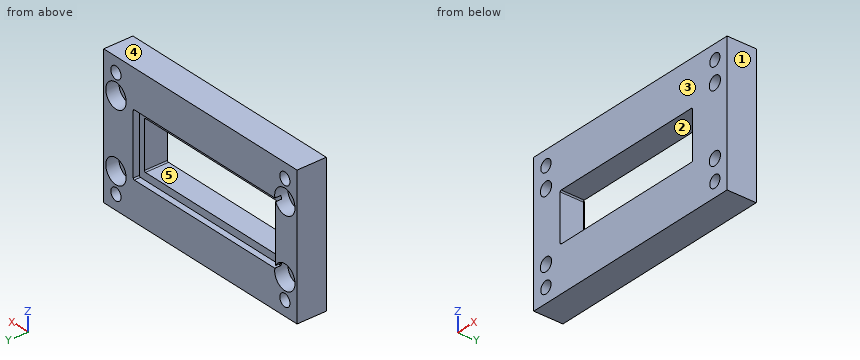
from build123d import *

# Parameters (mm, degrees)
SKETCH1_W                                   = 95
SKETCH1_H                                   = 57
SKETCH1_R                                   = 2.057983022
BOSS_EXTRUDE2_DEPTH                         = 12
BOSS_EXTRUDE3_DEPTH                         = 9.5
CBORE_FOR_M6_CHEESE_HEAD_SCREW1_D           = 5.5
CBORE_FOR_M6_CHEESE_HEAD_SCREW1_CBORE_D     = 10
CBORE_FOR_M6_CHEESE_HEAD_SCREW1_CBORE_DEPTH = 5.4
F_5_0_5_DIAMETER_HOLE1_D                    = 5


with BuildPart() as part:
    # Sketch1 → Boss-Extrude2 (new body)
    with BuildSketch(Plane(origin=(0, 0, 0), x_dir=(1, 0, 0), z_dir=(0, 1, 0))):
        Rectangle(SKETCH1_W, SKETCH1_H)
        with Locations(Location((41.5, 22.5, 0), (0, 0, 270))):
            Circle(SKETCH1_R, mode=Mode.SUBTRACT)
        with Locations(Location((-41.5, 22.5, 0), (0, 0, 270))):
            Circle(SKETCH1_R, mode=Mode.SUBTRACT)
        with Locations(Location((41.5, -22.5, 0), (0, 0, 270))):
            Circle(SKETCH1_R, mode=Mode.SUBTRACT)
        with Locations(Location((-41.5, -22.5, 0), (0, 0, 270))):
            Circle(SKETCH1_R, mode=Mode.SUBTRACT)
        with BuildLine():
            Line((-37, 12.5), (-37, -12.5))
            ThreePointArc((-37, -12.5), (-36.853553391, -12.853553391), (-36.5, -13))
            Line((-36.5, -13), (32.5, -13))
            ThreePointArc((32.5, -13), (32.853553391, -12.853553391), (33, -12.5))
            Line((33, -12.5), (33, 12.5))
            ThreePointArc((33, 12.5), (32.853553391, 12.853553391), (32.5, 13))
            Line((32.5, 13), (-36.5, 13))
            ThreePointArc((-36.5, 13), (-36.853553391, 12.853553391), (-37, 12.5))
        make_face(mode=Mode.SUBTRACT)
    extrude(amount=BOSS_EXTRUDE2_DEPTH)

    # Sketch1_5 → Boss-Extrude3 (add)
    with BuildSketch(Plane(origin=(0, 0, 0), x_dir=(1, 0, 0), z_dir=(0, 1, 0))):
        with BuildLine():
            ThreePointArc((-37, 12.5), (-36.853553391, 12.853553391), (-36.5, 13))
            Line((-36.5, 13), (32.5, 13))
            ThreePointArc((32.5, 13), (32.853553391, 12.853553391), (33, 12.5))
            Line((33, 12.5), (33, -12.5))
            ThreePointArc((33, -12.5), (32.853553391, -12.853553391), (32.5, -13))
            Line((32.5, -13), (-36.5, -13))
            ThreePointArc((-36.5, -13), (-36.853553391, -12.853553391), (-37, -12.5))
            Line((-37, -12.5), (-37, 12.5))
        make_face()
        with BuildLine():
            ThreePointArc((30, -10), (30.353553391, -9.853553391), (30.5, -9.5))
            Line((30.5, -9.5), (30.5, 9.5))
            ThreePointArc((30.5, 9.5), (30.353553391, 9.853553391), (30, 10))
            Line((30, 10), (-34, 10))
            ThreePointArc((-34, 10), (-34.353553391, 9.853553391), (-34.5, 9.5))
            Line((-34.5, 9.5), (-34.5, -9.5))
            ThreePointArc((-34.5, -9.5), (-34.353553391, -9.853553391), (-34, -10))
            Line((-34, -10), (30, -10))
        make_face(mode=Mode.SUBTRACT)
    extrude(amount=BOSS_EXTRUDE3_DEPTH)

    # CBORE for M6 Cheese Head Screw1 (through all)
    with Locations(Plane(origin=(-41.5, 12, -14), x_dir=(0, 0, 1), z_dir=(0, 1, 0))):
        with Locations((0, 0), (0, 83), (28, 83), (28, 0)):
            CounterBoreHole(CBORE_FOR_M6_CHEESE_HEAD_SCREW1_D / 2, CBORE_FOR_M6_CHEESE_HEAD_SCREW1_CBORE_D / 2, CBORE_FOR_M6_CHEESE_HEAD_SCREW1_CBORE_DEPTH)

    # 5.0 _5_ Diameter Hole1 (through all)
    with Locations(Plane(origin=(-41.5, 12, -22.5), x_dir=(0, 0, 1), z_dir=(0, 1, 0))):
        with Locations((0, 0), (0, 83), (45, 83), (45, 0)):
            Hole(F_5_0_5_DIAMETER_HOLE1_D / 2)


solid = part.part
The listing builds one solid part. Answer for the finished solid, in the listing's coordinates (mm). Face numbers are marked on the shaded views. A direction names the side the tool comes from. Give positions to 0.01 mm unless a question says otherwise; leave off trailing zeros. Write each loop counter-clockwise with the first axis right and the second up, starting at its lowest first coordinate (ties: lowest second). Pieces come first, ordered by that corner, then holes. Notation, with made-up numbers: (6, 53) - (46, 53) arc R14 ccw to (46, 79) - close; hole circle Ø8 at (6.5, 7.5). An arc over 180 degrees is marked (long way). Use a Markdown table: item, result.
1. Section D-D on x = -3.5 is taken. Write down the section's boundary in (y, z).
Values follow:
| item | result |
|---|---|
| outline | (0, -28.5) - (12, -28.5) - (12, -13) - (9.5, -13) - (9.5, -10) - (0, -10) - close; (0, 10) - (9.5, 10) - (9.5, 13) - (12, 13) - (12, 28.5) - (0, 28.5) - close |
2. Each of these flat-tipped pins is pushed along its axis until it touches: P1, Ø7, axis at x = -41.5, z = -14, coming from the -Y side; P2, Ø8, axis at x = 41.5, z = 14, coming from the +Y side. Where does it stop, or does it pass through?
Values follow:
| item | result |
|---|---|
| P1 | stops at y = 0 |
| P2 | stops at y = 6.6 |
3. Section A-A on z = -22.5 is taken. Write down the section's boundary in (x, y), plus the area to 3 significant figures.
Values follow:
| item | result |
|---|---|
| outline | (-47.5, 0) - (-44, 0) - (-44, 12) - (-47.5, 12) - close; (-39, 0) - (39, 0) - (39, 12) - (-39, 12) - close; (44, 0) - (47.5, 0) - (47.5, 12) - (44, 12) - close |
| area | 1,020 mm² |
4. For a pull along X with two mould halves and no side action, classify the marked faces 1, 2 and 3 as released by +X, released by -X, zero draft, split by the parting line, or undercut.
Values follow:
| item | result |
|---|---|
| face 1 | released by +X |
| face 2 | undercut |
| face 3 | zero draft |
5. Find the intervals of material crossed by probe 1 along X at (y, z) = (6.25, 22.5); probe 2 along X at (y, z) = (8.1, 14); probe 3 along Z at (x, y) = (-33, 8), in increasing order. Write a range as from..to.
Values follow:
| item | result |
|---|---|
| probe 1 | x = -47.5..-44, -39..39, 44..47.5 |
| probe 2 | x = -47.5..-46.5, -36.5..36.5, 46.5..47.5 |
| probe 3 | z = -28.5..-10, 10..28.5 |
6. Section C-C on y = 1.25 is taken. Count the separate pieces of the cut face and the enclosed holes in it, plus the area to 3 significant figures.
Values follow:
| item | result |
|---|---|
| separate pieces | 1 |
| enclosed holes | 9 |
| area | 3,940 mm² |
7. Section B-B on x = -41.5 is taken. Write down the section's boundary in (y, z).
Values follow:
| item | result |
|---|---|
| outline | (0, -28.5) - (12, -28.5) - (12, -25) - (0, -25) - close; (0, -20) - (12, -20) - (12, -19) - (6.6, -19) - (6.6, -16.75) - (0, -16.75) - close; (0, -11.25) - (6.6, -11.25) - (6.6, -9) - (12, -9) - (12, 9) - (6.6, 9) - (6.6, 11.25) - (0, 11.25) - close; (0, 16.75) - (6.6, 16.75) - (6.6, 19) - (12, 19) - (12, 20) - (0, 20) - close; (0, 25) - (12, 25) - (12, 28.5) - (0, 28.5) - close |
8. A tool of negligible diameter and unlimited length cuts with its end or side. For the marked faces 4 and 5, from which of +Z, -Z, +X, -X, +Y, -Y can it reach the whole face along a straight path? Write none if from no direction.
Values follow:
| item | result |
|---|---|
| face 4 | +Z, +X, -X, +Y, -Y |
| face 5 | +Y, -Y |
